Source: CAD feature listing. Evaluate the final solid. Frame: model axes, mm. A direction names the side the tool comes from. Coordinates: 2 decimals unless noted, no trailing zeros. Order: outer loops, then holes, each group sorted by start corner. A loop starts at its lowest first (then second) coordinate and runs counter-clockwise, first axis right, second up.
```python
from build123d import *

# Parameters (mm, degrees)
F0_R     = 25
F1_DEPTH = 10
F4_DEPTH = 8
F5_R     = 5


# Not quite as in the source:
# - a fillet or chamfer that OpenCascade refuses, or shapes differently, is made with other operations: its cross-section is extruded or revolved along the edge and cut away or added


with BuildPart() as f1:
    # F0 (on Top) → F1 (new body)
    with BuildSketch(Plane.XY):
        Circle(F0_R)
        Polygon((-18.8114806731, -6.112220586), (-11.6261344347, 16.0020012408), (11.6261344347, 16.0020012408), (18.8114806731, -6.112220586), (0, -19.7795613097), align=None, mode=Mode.SUBTRACT)
    extrude(amount=F1_DEPTH)

    # F2: fillet of radius 8 on 1 edges, made by hand

    # F2_s1 → F2_t2 (revolve, cut)
    with BuildSketch(Plane.XZ):
        with BuildLine():
            ThreePointArc((25, 2), (22.6568542495, 7.6568542495), (17, 10))
            Line((17, 10), (25, 10))
            Line((25, 10), (25, 2))
        make_face()
    revolve(axis=Axis((0, 0, 10), (0, 0, 1)), mode=Mode.SUBTRACT)

    # F3 (on Top) → F4 (join)
    with BuildSketch(Plane.XY):
        Polygon((6.539323839, 3.3114300304), (0, 0), (11.5929096937, -13.7071507052), (18.5771044344, 9.4072083011), align=None)
        Polygon((-6.539323839, 3.3114300304), (0, 0), (6.539323839, 3.3114300304), (0, 16.2251126021), align=None)
        Polygon((-11.5929096937, -13.7071507052), (0, 0), (-6.539323839, 3.3114300304), (-18.5771044344, 9.4072083011), align=None)
    extrude(amount=F4_DEPTH)

    # F5
    f5_edges = [f1.edges().sort_by_distance(p)[0] for p in [
        (-0.112981, 16.002001, 4),
        (0.112981, 16.002001, 4),
    ]]
    fillet(f5_edges, radius=F5_R)


solid = f1.part
```
1. Material intervals for line 1 along X through (y, z) = (14, 5.25); line 2 along Y through (x, z) = (8.5, 3); line 3 along Y through (x, z) = (8, 4.75), sorted ascending.
2. Access query for faces 1 (the flat face through (-10.438, 5.286, 3.944)), 2 (the flat face through (-16, 5, 10)), 3 (the flat face through (-0.2, 16.002, 8.3)). Directions: +Z, -Z, +X, -X, +Y, -Y. A direction counts if a zero-diameter tool reaches every point of the face in a straight line with its end or side. Return the directions, or none.
3. Section query B-B, the plane y = 6. Count the separate pieces of the cut face and the enclosed holes in it, plus the area to 3 significant figures.
4. Contact query for flat-ended pins moving along their axis: P1, Ø14, axis at x = -7.5, y = -4, coming from the +Z side; P2, Ø1.5, axis at y = -6, z = 6.5, coming from the -X side; P3, Ø4, axis at y = -5, z = 8, coming from the -X side. Output: stop coordinate, or through.
5. Section query A-A, the plane z = 7. Output: boundary loops of the cut face in (x, y) (3 decimals), plus the area to 3 significant figures.
Answer key:
1. line 1: x = -19.87 to -12.28, -4.25 to 4.25, 12.28 to 19.87
1. line 2: y = -23.44 to -13.6, -10.05 to 4.3, 16 to 23.44
1. line 3: y = -23.17 to -13.97, -9.46 to 4.05, 16 to 23.17
2. face 1: +Z, -Z
2. face 2: +Z, +X, -X, +Y, -Y
2. face 3: +Z
3. separate pieces: 3
3. enclosed holes: 0
3. area: 291 mm2
4. P1: stops at z = 8
4. P2: stops at x = -23.35
4. P3: stops at x = -23.47
5. outline: circle Ø46.49 at (0, 0); hole (-18.811, -6.112) - (-12.503, -10.696) - (-16.26, 1.74) - close; hole (-14.448, 7.316) - (-6.539, 3.311) - (-3.789, 8.743) arc R5 ccw to (-8.249, 16.002) - (-11.626, 16.002) - close; hole (-10.362, -12.251) - (0, -19.78) - (10.362, -12.251) - (0, 0) - close; hole (3.789, 8.743) - (6.539, 3.311) - (14.448, 7.316) - (11.626, 16.002) - (8.249, 16.002) arc R5 ccw to start; hole (12.503, -10.696) - (18.811, -6.112) - (16.26, 1.74) - close
5. area: 1,240 mm2
